Job drawing, mm, ordinate dimensions from the low corner. One solid piece. A direction names the side the tool comes from. Give positions to 0.01 mm unless a question says otherwise; leave off trailing zeros. Write each loop counter-clockwise with the first axis right and the second up, starting at its lowest first coordinate (ties: lowest second). Pieces come first, ordered by that corner, then holes. Notation, with made-up numbers: M 1,83.5 L 48,83.5 A20 cw 48,110.5 Z; hole C 88,54.25 d2. An arc over 180 degrees is marked long. Use a Markdown table: item, result.
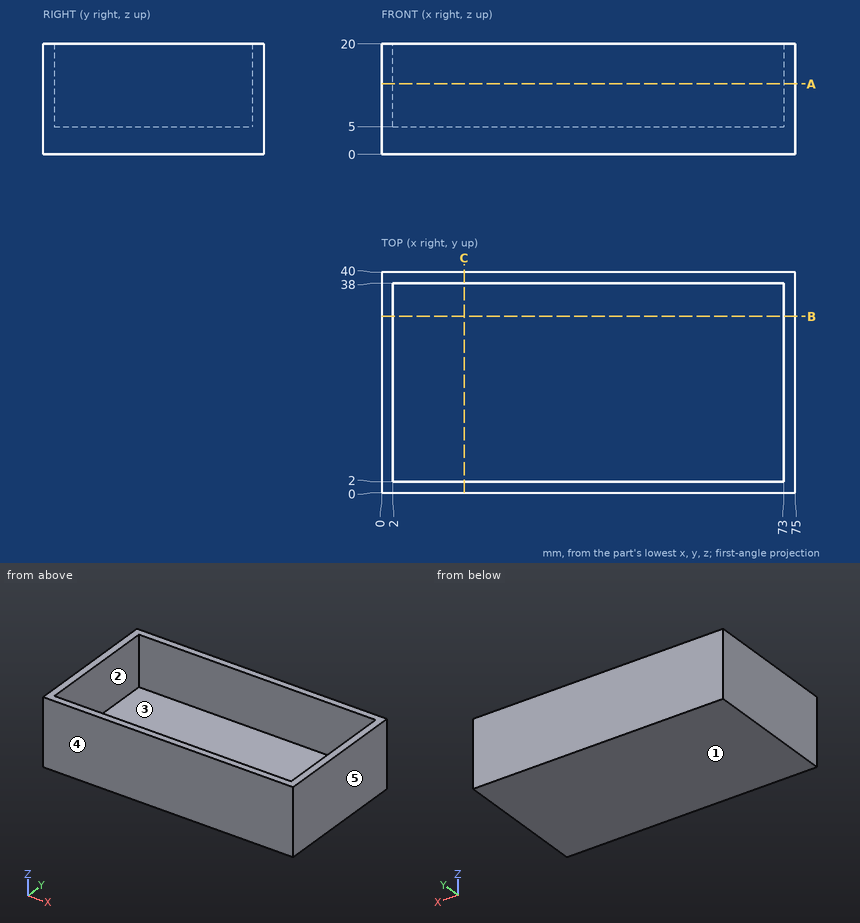
1. Drill centre lines: L1, parallel to Y at x = 66, z = 5.25; L2, parallel to X at y = 22, z = 18.5; L3, parallel to Z at x = 32, y = 21. Where is each one in solid material? Low to high.
Findings below:
| item | result |
|---|---|
| L1 | 0 to 2, 38 to 40 |
| L2 | 0 to 2, 73 to 75 |
| L3 | 0 to 5 |
2. Cut at B-B, the plane y = 32. Give the cut face in (x, z), then the cut area to 3 significant figures.
Findings below:
| item | result |
|---|---|
| outline | M 0,0 L 75,0 L 75,20 L 73,20 L 73,5 L 2,5 L 2,20 L 0,20 Z |
| area | 435 mm2 |
3. Cut at C-C, the plane x = 15. Give the cut face in (y, z).
Findings below:
| item | result |
|---|---|
| outline | M 0,0 L 40,0 L 40,20 L 38,20 L 38,5 L 2,5 L 2,20 L 0,20 Z |
4. Tool access for the marked faces 1 and 2: list every direction of +Z, -Z, +X, -X, +Y, -Y with a clear straight run to the whole face (end or side of a thin tool).
Findings below:
| item | result |
|---|---|
| face 1 | -Z, +X, -X, +Y, -Y |
| face 2 | +Z |
5. Two-plate mould, pull along Y, no slides. Class the marked faces 3, 4 and 5: released by +Y, released by -Y, zero draft, split by the parting line, or undercut.
Findings below:
| item | result |
|---|---|
| face 3 | undercut |
| face 4 | released by -Y |
| face 5 | zero draft |
6. Cut at A-A, the plane z = 12.75. Give the cut face in (x, y), then the cut area to 3 significant figures.
Findings below:
| item | result |
|---|---|
| outline | M 0,0 L 75,0 L 75,40 L 0,40 Z; hole M 2,2 L 73,2 L 73,38 L 2,38 Z |
| area | 444 mm2 |
7. Drop a flat-ended pin along its axis: P1, Ø2, axis at x = 40, y = 21, coming from the -Z side. Give the stop position or say it passes through.
Findings below:
| item | result |
|---|---|
| P1 | z = 0 |
